```python
from build123d import *

# Parameters (mm, degrees)
SKETCH_1_W               = 45.5
SKETCH_1_H               = 45.5
EXTRUDE_1_DEPTH          = 370
CUT_EXTRUDE_1_REACH      = 380.964
SKETCH_2_W               = 8
SKETCH_2_H               = 8
MIRROR_2_COPY_1_REACH    = 380.964
MIRROR_2_COPY_1_SKETCH_W = 8
MIRROR_2_COPY_1_SKETCH_H = 8
CUT_EXTRUDE_2_REACH      = 380.964
MIRROR_4_COPY_1_REACH    = 380.964
FILLET_1_R               = 2
CUT_EXTRUDE_4_REACH      = 380.964
SKETCH_6_R               = 5


with BuildPart() as part:
    # Sketch 1 → Extrude 1 (new body)
    with BuildSketch(Plane(origin=(0, 0, 0), x_dir=(0, 0, -1), z_dir=(1, 0, 0))):
        with Locations((37.954960836, 32.285758607)):
            Rectangle(SKETCH_1_W, SKETCH_1_H)
    extrude(amount=EXTRUDE_1_DEPTH)

    # Sketch 2 → Cut-Extrude 1 (cut, up to next)
    with BuildSketch(Plane(origin=(370, 0, 0), x_dir=(0, 0, -1), z_dir=(1, 0, 0)), mode=Mode.PRIVATE) as cut_extrude_1_sk1:
        Polygon((31.804960836, 55.035758607), (31.804960836, 54.035758607), (32.804960836, 54.035758607), (32.804960836, 50.505758607), (30.174960836, 50.505758607), (30.174960836, 52.505758607), (26.774960836, 52.505758607), (26.774960836, 45.005758607), (30.454960836, 41.905758607), (37.954960836, 41.905758607), (37.954960836, 55.035758607), align=None)
    cut_extrude_1_tool1 = extrude(cut_extrude_1_sk1.sketch, amount=-CUT_EXTRUDE_1_REACH, mode=Mode.PRIVATE) & part.part
    # Sketch 2 → Cut-Extrude 1 (cut, up to next)
    with BuildSketch(Plane(origin=(370, 0, 0), x_dir=(0, 0, -1), z_dir=(1, 0, 0)), mode=Mode.PRIVATE) as cut_extrude_1_sk2:
        with Locations((20.604960836, 49.635758607)):
            Rectangle(SKETCH_2_W, SKETCH_2_H)
    cut_extrude_1_tool2 = extrude(cut_extrude_1_sk2.sketch, amount=-CUT_EXTRUDE_1_REACH, mode=Mode.PRIVATE) & part.part
    cut_extrude_1_1 = cut_extrude_1_tool1.solids().sort_by_distance((370, 47.983788, -32.930174))[0]
    add(cut_extrude_1_1, mode=Mode.SUBTRACT)
    cut_extrude_1_2 = cut_extrude_1_tool2.solids().sort_by_distance((370, 49.635759, -20.604961))[0]
    add(cut_extrude_1_2, mode=Mode.SUBTRACT)
    cut_extrude_1 = cut_extrude_1_1 + cut_extrude_1_2  # Cut-Extrude 1 as one shape, for the pattern or mirror that repeats it

    # Mirror 1: Cut-Extrude 1 across plane
    add(cut_extrude_1.mirror(Plane(origin=(0, 0, -37.954960836), x_dir=(1, 0, 0), z_dir=(0, 0, -1))), mode=Mode.SUBTRACT)

    # Mirror 2: Cut-Extrude 1 across plane
    add(cut_extrude_1.mirror(Plane(origin=(0, 32.285758607, 0), x_dir=(0, 0, 1), z_dir=(0, -1, 0))), mode=Mode.SUBTRACT)

    # Mirror 2 copy 1 sketch → Mirror 2 copy 1 (cut, up to next)
    with BuildSketch(Plane(origin=(370, 64.571517214, -75.909921671), x_dir=(0, 0, 1), z_dir=(1, 0, 0)), mode=Mode.PRIVATE) as mirror_2_copy_1_sk1:
        Polygon((31.804960836, 55.035758607), (31.804960836, 54.035758607), (32.804960836, 54.035758607), (32.804960836, 50.505758607), (30.174960836, 50.505758607), (30.174960836, 52.505758607), (26.774960836, 52.505758607), (26.774960836, 45.005758607), (30.454960836, 41.905758607), (37.954960836, 41.905758607), (37.954960836, 55.035758607), align=None)
    mirror_2_copy_1_tool1 = extrude(mirror_2_copy_1_sk1.sketch, amount=-MIRROR_2_COPY_1_REACH, mode=Mode.PRIVATE) & part.part
    # Mirror 2 copy 1 sketch → Mirror 2 copy 1 (cut, up to next)
    with BuildSketch(Plane(origin=(370, 64.571517214, -75.909921671), x_dir=(0, 0, 1), z_dir=(1, 0, 0)), mode=Mode.PRIVATE) as mirror_2_copy_1_sk2:
        with Locations((20.604960836, 49.635758607)):
            Rectangle(MIRROR_2_COPY_1_SKETCH_W, MIRROR_2_COPY_1_SKETCH_H)
    mirror_2_copy_1_tool2 = extrude(mirror_2_copy_1_sk2.sketch, amount=-MIRROR_2_COPY_1_REACH, mode=Mode.PRIVATE) & part.part
    add(mirror_2_copy_1_tool1.solids().sort_by_distance((370, 16.587729214, -42.979747671))[0], mode=Mode.SUBTRACT)
    add(mirror_2_copy_1_tool2.solids().sort_by_distance((370, 14.935758214, -55.304960671))[0], mode=Mode.SUBTRACT)

    # Sketch 3 → Cut-Extrude 2 (cut, up to next)
    with BuildSketch(Plane(origin=(370, 0, 0), x_dir=(0, 0, -1), z_dir=(1, 0, 0)), mode=Mode.PRIVATE) as cut_extrude_2_sk1:
        Polygon((15.204960836, 38.435758607), (16.204960836, 38.435758607), (16.204960836, 37.435758607), (19.734960836, 37.435758607), (19.734960836, 40.065758607), (17.734960836, 40.065758607), (17.734960836, 43.465758607), (25.234960836, 43.465758607), (28.534960836, 39.785758607), (28.534960836, 32.285758607), (15.204960836, 32.285758607), align=None)
    cut_extrude_2_tool1 = extrude(cut_extrude_2_sk1.sketch, amount=-CUT_EXTRUDE_2_REACH, mode=Mode.PRIVATE) & part.part
    cut_extrude_2 = cut_extrude_2_tool1.solids().sort_by_distance((370, 37.306091, -22.347242))[0]
    add(cut_extrude_2, mode=Mode.SUBTRACT)

    # Mirror 3: Cut-Extrude 2 across plane
    add(cut_extrude_2.mirror(Plane(origin=(0, 32.285758607, 0), x_dir=(0, 0, 1), z_dir=(0, -1, 0))), mode=Mode.SUBTRACT)

    # Mirror 4: Cut-Extrude 2 across plane
    add(cut_extrude_2.mirror(Plane(origin=(0, 0, -37.954960836), x_dir=(1, 0, 0), z_dir=(0, 0, -1))), mode=Mode.SUBTRACT)

    # Mirror 4 copy 1 sketch → Mirror 4 copy 1 (cut, up to next)
    with BuildSketch(Plane(origin=(370, 64.571517214, -75.909921671), x_dir=(0, 0, 1), z_dir=(1, 0, 0)), mode=Mode.PRIVATE) as mirror_4_copy_1_sk1:
        Polygon((15.204960836, 38.435758607), (16.204960836, 38.435758607), (16.204960836, 37.435758607), (19.734960836, 37.435758607), (19.734960836, 40.065758607), (17.734960836, 40.065758607), (17.734960836, 43.465758607), (25.234960836, 43.465758607), (28.534960836, 39.785758607), (28.534960836, 32.285758607), (15.204960836, 32.285758607), align=None)
    mirror_4_copy_1_tool1 = extrude(mirror_4_copy_1_sk1.sketch, amount=-MIRROR_4_COPY_1_REACH, mode=Mode.PRIVATE) & part.part
    add(mirror_4_copy_1_tool1.solids().sort_by_distance((370, 27.265426214, -53.562679671))[0], mode=Mode.SUBTRACT)

    # Fillet 1
    fillet_1_edges = [part.edges().sort_by_distance(p)[0] for p in [
        (185, 55.035758607, -15.204960836),
        (185, 55.035758607, -60.704960836),
        (185, 9.535758607, -60.704960836),
        (185, 9.535758607, -15.204960836),
    ]]
    fillet(fillet_1_edges, radius=FILLET_1_R)

    # Sketch 6 → Cut-Extrude 4 (cut, up to next)
    with BuildSketch(Plane(origin=(370, 0, 0), x_dir=(0, 0, -1), z_dir=(1, 0, 0)), mode=Mode.PRIVATE) as cut_extrude_4_sk1:
        with Locations((37.954960836, 32.285758607)):
            Circle(SKETCH_6_R)
    cut_extrude_4_tool1 = extrude(cut_extrude_4_sk1.sketch, amount=-CUT_EXTRUDE_4_REACH, mode=Mode.PRIVATE) & part.part
    add(cut_extrude_4_tool1.solids().sort_by_distance((370, 32.285759, -37.954961))[0], mode=Mode.SUBTRACT)


solid = part.part
```
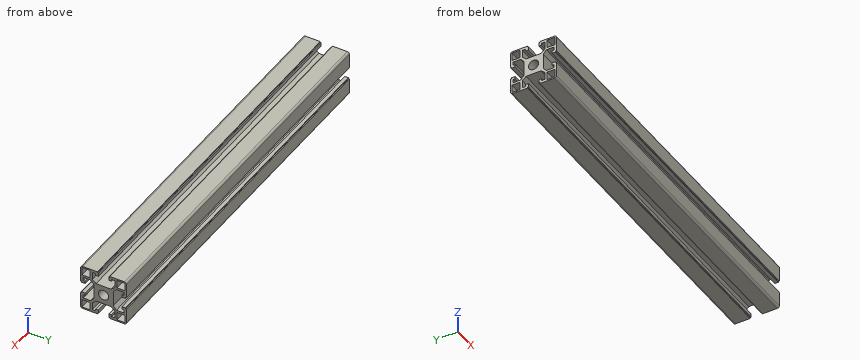
Part model, mm, in its own coordinate system. Give positions to 0.01 mm unless a question says otherwise; leave off trailing zeros. Use CSV: the item, a comma, the result in double quotes.
Item 1: Drill centre lines: probe 1 along Y at (x, z) = (230.5, -51.5); probe 2 along Y at (x, z) = (272, -45.5); probe 3 along Y at (x, z) = (242, -57). Where is each one in solid material? Low to high.
Taken from the geometry:
probe 1,"y = 9.54 to 10.94, 18.94 to 21.11, 43.47 to 45.64, 53.64 to 55.04"
probe 2,"y = 9.54 to 14.07, 22.63 to 41.94, 50.51 to 55.04"
probe 3,"y = 9.54 to 10.94, 18.94 to 21.11, 24.51 to 27.14, 37.44 to 40.07, 43.47 to 45.64, 53.64 to 55.04"
Item 2: Slice it at A-A on x = 39.5. State how many separate pieces and enclosed holes the cut face has, plus the area to 3 significant figures.
Taken from the geometry:
separate pieces,"1"
enclosed holes,"5"
area,"752 mm²"
Item 3: Pin check, flat tips, straight feed: P1, Ø0.5, axis at x = 235, y = 38, coming from the +Z side; P2, Ø12, axis at y = 45.5, z = -36.5, coming from the +X side; P3, Ø1.1, axis at x = 121, z = -32.5, coming from the +Y side; P4, Ø0.8, axis at x = 252, y = 54.5, coming from the -Z side. Stop position of each tip, or through.
Taken from the geometry:
P1,"stops at z = -16.2"
P2,"stops at x = 370"
P3,"stops at y = 54.04"
P4,"stops at z = -60.4"
